```python
from build123d import *

# Parameters (mm, degrees)
F0_W      = 33
F0_H      = 3.825
F1_DEPTH  = 10
F2_R      = 1.75
F3_DEPTH  = 16.651
F4_W      = 18
F4_H      = 3.4
F4_W_2    = 2.75
F4_H_2    = 6
F5_DEPTH  = 12.151
F6_R      = 1.75
F7_DEPTH  = 15
F10_DEPTH = 2
F11_W     = 17.65
F11_H     = 60
F12_DEPTH = 8
F13_R     = 1.75
F14_DEPTH = 63.001
F15_R     = 2.75
F15_R_2   = 1.75
F16_DEPTH = 0.3
F17_R     = 1.75
F18_DEPTH = 2
F19_R     = 3.75
F20_DEPTH = 4


# Not quite as in the source:
# - a pattern or mirror of a feature is missing from the dataset's text; its kind, count and spacing are read off the source's solid


with BuildPart() as f1:
    # F0 (on Top) → F1 (new body)
    with BuildSketch(Plane.XY):
        Polygon((0, -3.825), (0, 0), (-3, 0), (-3, -4.6), (-15, -4.6), (-15, -8.325), (0, -8.325), align=None)
        Polygon((-3, 0), (0, 0), (0, 3.825), (0, 8.325), (-15, 8.325), (-15, 4.6), (-3, 4.6), align=None)
        with Locations((16.5, 1.9125)):
            Rectangle(F0_W, F0_H)
        with Locations((16.5, -1.9125)):
            Rectangle(F0_W, F0_H)
    extrude(amount=F1_DEPTH)

    # F2 (on face) → F3 (cut, through all)
    with BuildSketch(Plane.XZ.offset(8.325)):
        with Locations((-9.9527407438, 5)):
            Circle(F2_R)
    extrude(amount=-F3_DEPTH, mode=Mode.SUBTRACT)

    # F4 (on face) → F5 (cut, through all)
    with BuildSketch(Plane.XZ.offset(3.825)):
        with Locations((12.4002694301, 5)):
            Rectangle(F4_W, F4_H)
        with Locations((28.125, 5)):
            Rectangle(F4_W_2, F4_H_2)
    extrude(amount=-F5_DEPTH, mode=Mode.SUBTRACT)

    # F6 (on face) → F7 (cut)
    with BuildSketch(Plane.YZ.offset(33)):
        with Locations((0, 5)):
            Circle(F6_R)
    extrude(amount=-F7_DEPTH, mode=Mode.SUBTRACT)

    # F15 (on face) → F16 (join)
    with BuildSketch(Plane.XZ.offset(-4.6)):
        with Locations((-9.9527407438, 5)):
            Circle(F15_R)
        with Locations((-9.9527407438, 5)):
            Circle(F15_R_2, mode=Mode.SUBTRACT)
    f16 = extrude(amount=F16_DEPTH)

    # F16_copies: F16 across plane
    add(f16.mirror(Plane(origin=(0, 0, 0), x_dir=(0, 0, -1), z_dir=(0, -1, 0))))

    # F17 (on face) → F18 (cut)
    with BuildSketch(Plane.XZ.offset(8.325)):
        Polygon((-7.9284293953, 1.9088033227), (-6.2635302189, 5.2075067143), (-8.2878415673, 8.2987033916), (-11.9770520922, 8.0911966773), (-13.6419512686, 4.7924932857), (-11.6176399202, 1.7012966084), align=None)
        with Locations((-9.9527407438, 5)):
            Circle(F17_R, mode=Mode.SUBTRACT)
    f18 = extrude(amount=-F18_DEPTH, mode=Mode.SUBTRACT)

    # F18_copies: F18 across plane
    add(f18.mirror(Plane.ZX), mode=Mode.SUBTRACT)


with BuildPart() as f10:
    # F9 (on offset) → F10 (new body)
    with BuildSketch(Plane.YZ.offset(38)):
        Polygon((3.825, 0), (3.825, 10), (3.825, 19.8484882712), (-3.825, 19.8484882712), (-3.825, 10), (-3.825, 0), (-3.825, -10.1515117288), (3.825, -10.1515117288), align=None)
    extrude(amount=F10_DEPTH)

    # F11 (on face) → F12 (join)
    with BuildSketch(Plane.YZ.offset(40)):
        with Locations((0, 4.8484882712)):
            Rectangle(F11_W, F11_H)
    extrude(amount=F12_DEPTH)

    # F13 (on face) → F14 (cut, through all)
    with BuildSketch(Plane.YZ.offset(48)):
        with Locations((0, 5)):
            Circle(F13_R)
    extrude(amount=-F14_DEPTH, mode=Mode.SUBTRACT)

    # F19 (on face) → F20 (join)
    with BuildSketch(Plane(origin=(40, 0, 0), x_dir=(0, -1, 0), z_dir=(-1, 0, 0))):
        with Locations((0, 28)):
            Circle(F19_R)
        with Locations((0, -18)):
            Circle(F19_R)
    extrude(amount=F20_DEPTH)


solid = f1.part
```
Build history of the part. All positions in model axes, mm. A direction names the side the tool comes from. Coordinates: 2 decimals unless noted, no trailing zeros. Order: outer loops, then holes, each group sorted by start corner. A loop starts at its lowest first (then second) coordinate and runs counter-clockwise, first axis right, second up.
Item 1: Saw through at D-D on y = 0. List the corners of the cut face in (x, z).
Filled in:
outline: (-3, 0) - (33, 0) - (33, 3.25) - (29.5, 3.25) - (29.5, 2) - (26.75, 2) - (26.75, 3.25) - (18, 3.25) - (18, 3.3) - (3.4, 3.3) - (3.4, 6.7) - (18, 6.7) - (18, 6.75) - (26.75, 6.75) - (26.75, 8) - (29.5, 8) - (29.5, 6.75) - (33, 6.75) - (33, 10) - (-3, 10) - close
Item 2: Drill centre lines: L1, parallel to X at y = 2, z = 5.25; L2, parallel to X at y = 3, z = 2.75; L3, parallel to Z at x = 24.5, y = 0. Where is each one in solid material? Low to high.
Filled in:
L1: x = -3 to 3.4, 21.4 to 26.75, 29.5 to 33
L2: x = -3 to 26.75, 29.5 to 33
L3: z = 0 to 3.25, 6.75 to 10
Item 3: Mould opens along Z. For faces 1 (the flat face through (9, 0, 10)), 2 (the flat face through (33, -2, 5)), 3 (the flat face through (-10.107, 7.339, 8.196)) say: released by +Z, released by -Z, zero draft, split by the parting line, or undercut.
Filled in:
face 1: released by +Z
face 2: zero draft
face 3: undercut
Item 4: Drop flat-ended pins along their axis: pin 1 Ø3.5 at (y, z) = (-2.5, 6) entering from -X; pin 2 Ø1.7 at (y, z) = (0, 5.5) entering from +X; pin 3 Ø3 at (x, z) = (-10.5, 5) entering from +Y (3 decimals). Give the stop position or say it passes through.
Filled in:
pin 1: stops at x = -3
pin 2: stops at x = 3.4
pin 3: stops at y = 6.325
Item 5: Saw through at B-B on y = 2.75. List the corners of the cut face in (x, z).
Filled in:
outline: (-3, 0) - (33, 0) - (33, 10) - (-3, 10) - close; hole (3.4, 3.3) - (21.4, 3.3) - (21.4, 6.7) - (3.4, 6.7) - close; hole (26.75, 2) - (29.5, 2) - (29.5, 8) - (26.75, 8) - close
Item 6: Tool access for faces 4 (the flat face through (-12.644, 7.339, 3.269)), 5 (the cylindrical face through (23.41, -1.75, 5.08)), 6 (the flat face through (-10, -4.3, 3)), 7 (the flat face through (-9.799, -7.339, 1.804)): list every direction of +Z, -Z, +X, -X, +Y, -Y with a clear straight run to the whole face (end or side of a thin tool).
Filled in:
face 4: +Y
face 5: +X
face 6: +Z, -Z, -X
face 7: -Y
Item 7: Saw through at C-C on z = 9. List the corners of the cut face in (x, y) (3 decimals).
Filled in:
outline: (-15, -8.325) - (0, -8.325) - (0, -3.825) - (33, -3.825) - (33, 3.825) - (0, 3.825) - (0, 8.325) - (-15, 8.325) - (-15, 4.6) - (-3, 4.6) - (-3, -4.6) - (-15, -4.6) - close
Item 8: Saw through at A-A on x = 10. List the corners of the cut face in (y, z) (3 decimals).
Filled in:
outline: (-3.825, 0) - (3.825, 0) - (3.825, 3.3) - (-3.825, 3.3) - close; (-3.825, 6.7) - (3.825, 6.7) - (3.825, 10) - (-3.825, 10) - close
